Could you check a few things on this model? Use its own coordinates, in mm. Round coordinates to 2 decimals unless told otherwise and drop trailing zeros. Loops run counter-clockwise (first coordinate to the right, second up) from the corner with the lowest first, then second, coordinate; pieces in that order, holes last. Notation, with made-up numbers: (-22.75, -6.75) -> (17.25, -6.75) arc R19 ccw to (17.25, -2.75) -> close; hole circle Ø6 at (-28.5, -13.75). An arc over 180 degrees is marked (long way). One line per item, written item: value.
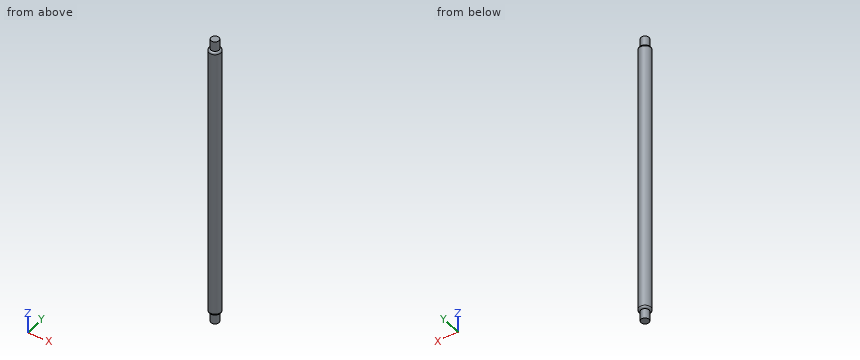
```python
from build123d import *

# Parameters (mm, degrees)
SKETCH1_R            = 6
BOSS_EXTRUDE1_DEPTH  = 150
SKETCH2_R            = 6
SKETCH2_R_2          = 4
CUT_EXTRUDE1_DEPTH   = 10
FILLET1_R            = 2
FILLET1_OF_MIRROR1_R = 2


with BuildPart() as part:
    # Sketch1 → Boss-Extrude1 (new, symmetric)
    with BuildSketch(Plane.XY):
        Circle(SKETCH1_R)
    extrude(amount=BOSS_EXTRUDE1_DEPTH, both=True)

    # Sketch2 → Cut-Extrude1 (cut)
    with BuildSketch(Plane.XY.offset(150)):
        Circle(SKETCH2_R)
        Circle(SKETCH2_R_2, mode=Mode.SUBTRACT)
    cut_extrude1 = extrude(amount=-CUT_EXTRUDE1_DEPTH, mode=Mode.SUBTRACT)

    # Fillet1
    fillet1_edges = [part.edges().sort_by_distance(p)[0] for p in [
        (-6, 0, 140),
    ]]
    fillet(fillet1_edges, radius=FILLET1_R - 0.0001)  # a hair under: the kernel refuses the full size

    # Mirror1: Cut-Extrude1 across plane
    add(cut_extrude1.mirror(Plane.XY), mode=Mode.SUBTRACT)

    # Fillet1 of Mirror1
    fillet1_of_mirror1_edges = [part.edges().sort_by_distance(p)[0] for p in [
        (-6, 0, -140),
    ]]
    fillet(fillet1_of_mirror1_edges, radius=FILLET1_OF_MIRROR1_R - 0.0001)  # a hair under: the kernel refuses the full size


solid = part.part
```
Item 1: I need wall thicknesses on line 1 (Y direction, x = -4.5, z = -94); line 2 (Y direction, x = -3.5, z = -106). Which ranges of each line are inside material? Lowest first, please. Write a range as from..to.
Output:
line 1: y = -3.97..3.97
line 2: y = -4.87..4.87
Item 2: Will these pins go through, and if not, where does the flat tip stop? pin 1 Ø2 at (y, z) = (-3, -103.5) entering from -X; pin 2 Ø3 at (x, z) = (-4.5, 6.5) entering from -Y; pin 3 Ø1 at (x, z) = (-3, 104) entering from +Y.
Output:
pin 1: stops at x = -5.66
pin 2: stops at y = -5.2
pin 3: stops at y = 5.45
Item 3: If we section it at C-C on z = -35.5: List the corners of the cut face in (x, y) for me, plus the area to 3 significant figures.
Output:
outline: circle Ø12 at (0, 0)
area: 113 mm²
